The model under review builds one solid part; all positions refer to its coordinate system, in mm. Coordinates: 2 decimals unless noted, no trailing zeros. Loops run counter-clockwise (first coordinate to the right, second up) from the corner with the lowest first, then second, coordinate; pieces in that order, holes last. Notation, with made-up numbers: M 17.5,-21 L 75.5,-21 A8 ccw 75.5,-14 Z; hole C 69,15.25 d1. An arc over 180 degrees is marked long. Return JSON: item names as keys, results as strings.
```python
from build123d import *

# Parameters (mm, degrees)
F0_W     = 66.183033
F0_H     = 87.93332
F1_DEPTH = 25.4
F2_R     = 13.013131
F3_DEPTH = 6.35
F4_DEPTH = 6.3754


with BuildPart() as f1:
    # F0 (on Top) → F1 (new body)
    with BuildSketch(Plane.XY):
        with Locations((-4.194698, 2.330387)):
            Rectangle(F0_W, F0_H)
    extrude(amount=F1_DEPTH)

    # F2 (on face) → F3 (join)
    with BuildSketch(Plane.XY.offset(25.4)):
        with Locations((0, -27.032504)):
            Circle(F2_R)
    extrude(amount=F3_DEPTH)

    # F2 (on face) → F4 (join)
    with BuildSketch(Plane.XY.offset(25.4)):
        with BuildLine():
            ThreePointArc((-1.99442, 46.297047), (2.81281, 17.061409), (27.629392, 33.246875))
            ThreePointArc((27.629392, 33.246875), (26.128457, 40.377055), (21.880402, 46.297047))
            Line((21.880402, 46.297047), (-1.99442, 46.297047))
        make_face()
    extrude(amount=F4_DEPTH)


solid = f1.part
```
1. The part is to be moulded in two halves that separate along Y. For faces 1 (the face through (-5, 3, 25.4)), 2 (the face through (-5, -41.636, 13)), 3 (the face through (-2.821, -39.736, 28.531)), 4 (the face through (0, -27, 31.75)), say which applies: released by +Y, released by -Y, zero draft, split by the parting line, or undercut.
Check values:
{"face 1": "undercut", "face 2": "released by -Y", "face 3": "undercut", "face 4": "zero draft"}
2. Add section B-B on y = -23. Give the boundary of the cut face in (x, z).
Check values:
{"outline": "M -37.29,0 L 28.9,0 L 28.9,25.4 L 12.37,25.4 L 12.37,31.75 L -12.37,31.75 L -12.37,25.4 L -37.29,25.4 Z"}
3. To check wall thickness, follow line 1 (Z direction, x = -28, y = -17.5); line 2 (Z direction, x = 1, y = -14.5); line 3 (X direction, y = 19, z = 30). State the ranges of each line that lie inside material, in increasing order.
Check values:
{"line 1": "0 to 25.4", "line 2": "0 to 31.75", "line 3": "-0.54 to 20.42"}
4. Insertion check: pin 1 Ø4 at (x, y) = (1.5, 4) entering from +Z; pin 2 Ø21 at (x, y) = (-3.5, -23) entering from +Z. Each pin has a flat end and moves straight along its axis. Give the tip position at first contact, or say it passes through.
Check values:
{"pin 1": "z = 25.4", "pin 2": "z = 31.75"}
5. Add section A-A on x = 0. Give the boundary of the cut face in (y, z), plus the area to 3 significant figures.
Check values:
{"outline": "M -41.64,0 L 46.3,0 L 46.3,31.78 L 18.62,31.78 L 18.62,25.4 L -14.02,25.4 L -14.02,31.75 L -40.05,31.75 L -40.05,25.4 L -41.64,25.4 Z", "area": "2,580 mm²"}
6. Add section D-D on y = 40. Give the boundary of the cut face in (x, z).
Check values:
{"outline": "M -37.29,0 L 28.9,0 L 28.9,25.4 L 26.29,25.4 L 26.29,31.78 L -6.4,31.78 L -6.4,25.4 L -37.29,25.4 Z"}
7. Add section C-C on x = -14.5. Give the boundary of the cut face in (y, z), plus the area to 3 significant figures.
Check values:
{"outline": "M -41.64,0 L 46.3,0 L 46.3,25.4 L -41.64,25.4 Z", "area": "2,230 mm²"}
